Work out the finished part from the listing and answer in its coordinate system (mm). A direction names the side the tool comes from. Give positions to 0.01 mm unless a question says otherwise; leave off trailing zeros. Loops run counter-clockwise (first coordinate to the right, second up) from the corner with the lowest first, then second, coordinate; pieces in that order, holes last. Notation, with made-up numbers: (57, -21.75) - (80, -21.75) arc R16 cw to (80, -6.75) - close; hole circle Ø9 at (74.5, -7). An arc over 180 degrees is marked (long way). Use CSV: the item, a comma, the result in double quotes.
from build123d import *

# Parameters (mm, degrees)
BOSS_EXTRUDE1_DEPTH = 11.5
SKETCH4_R           = 4.5
CUT_EXTRUDE2_DEPTH  = 5
SKETCH5_R           = 2.75
CUT_EXTRUDE3_DEPTH  = 89.726115198
SKETCH6_R           = 2.5
CUT_EXTRUDE4_DEPTH  = 50.330582837
CUT_EXTRUDE5_DEPTH  = 8.2
CUT_EXTRUDE6_DEPTH  = 9
FILLET1_R           = 5.05
FILLET2_R           = 5
BOSS_EXTRUDE2_DEPTH = 18
SKETCH3_R           = 2.5
CUT_EXTRUDE1_DEPTH  = 4


with BuildPart() as part:
    # Sketch1 → Boss-Extrude1 (new body)
    with BuildSketch(Plane(origin=(0, 0, 0), x_dir=(1, 0, 0), z_dir=(0, 1, 0))):
        with BuildLine():
            Line((48.493420768, -25), (75.993420768, -25))
            ThreePointArc((75.993420768, -25), (79.695575847, 6.97245942), (70.497705508, 37.816312856))
            Line((70.497705508, 37.816312856), (43.415492301, 33.04098797))
            ThreePointArc((43.415492301, 33.04098797), (54.350723514, 4.755072162), (48.493420768, -25))
        make_face()
    extrude(amount=BOSS_EXTRUDE1_DEPTH)

    # Sketch4 → Cut-Extrude2 (cut)
    with BuildSketch(Plane.XZ):
        with Locations(Location((73.026415161, 17, 0), (0, 0, 270))):
            Circle(SKETCH4_R)
        with Locations(Location((68.964960805, -29.422635715, 0), (0, 0, 270))):
            Circle(SKETCH4_R)
    extrude(amount=-CUT_EXTRUDE2_DEPTH, mode=Mode.SUBTRACT)

    # Sketch5 → Cut-Extrude3 (cut, through all)
    with BuildSketch(Plane.XZ.offset(-5)):
        with Locations(Location((73.026415161, 17, 0), (0, 0, 270))):
            Circle(SKETCH5_R)
        with Locations(Location((68.964960805, -29.422635715, 0), (0, 0, 270))):
            Circle(SKETCH5_R)
    extrude(amount=-CUT_EXTRUDE3_DEPTH, mode=Mode.SUBTRACT)

    # Sketch6 → Cut-Extrude4 (cut, through all)
    with BuildSketch(Plane(origin=(45.954456534, 0, -4.020493985), x_dir=(0.08715574274765857, 0, 0.9961946980917455), z_dir=(-0.9961946980917455, 0, 0.08715574274765857))):
        with Locations((0, 7.5)):
            Circle(SKETCH6_R)
    extrude(amount=-CUT_EXTRUDE4_DEPTH, mode=Mode.SUBTRACT)

    # Sketch8 → Cut-Extrude5 (cut)
    with BuildSketch(Plane(origin=(79.695575847, 0, -6.97245942), x_dir=(-0.08715574274765857, 0, -0.9961946980917455), z_dir=(0.9961946980917455, 0, -0.08715574274765857))):
        with BuildLine():
            Line((-4.5, 7.5), (-4.5, 11.5))
            Line((-4.5, 11.5), (4.5, 11.5))
            Line((4.5, 11.5), (4.5, 7.5))
            ThreePointArc((4.5, 7.5), (0, 3), (-4.5, 7.5))
        make_face()
    extrude(amount=-CUT_EXTRUDE5_DEPTH, mode=Mode.SUBTRACT)

    # Sketch7 → Cut-Extrude6 (cut)
    with BuildSketch(Plane(origin=(0, 11.5, 0), x_dir=(1, 0, 0), z_dir=(0, 1, 0))):
        Polygon((51.16274886, 9.5454507), (52.043021862, -0.516115751), (60.012579447, 0.181130191), (59.132306445, 10.242696642), align=None)
    extrude(amount=-CUT_EXTRUDE6_DEPTH, mode=Mode.SUBTRACT)

    # Fillet1
    # the kernel refuses this fillet: 5.05 mm, written as the material it adds along each edge
    with BuildSketch(Plane(origin=(41.980572745, 2.5, 1.396465976), x_dir=(0, 1, 0), z_dir=(0.9961946980917454, 0, -0.08715574274765918))) as fillet1_piece_1_section:
        with BuildLine():
            CenterArc((FILLET1_R, -FILLET1_R), FILLET1_R, 90, 90)
            Line((0, -FILLET1_R), (0, 0))
            Line((0, 0), (FILLET1_R, 0))
        make_face()
    fillet1_piece_1 = extrude(amount=30.725886038, mode=Mode.PRIVATE)
    fillet1_piece_1 = fillet1_piece_1 - Plane(origin=(0, 3.651800065, 0), x_dir=(0.7957627874759549, 0, -0.6056084428642803), z_dir=(0, -1, 0)) * Cylinder(54.558334448, 82, mode=Mode.PRIVATE)
    add(fillet1_piece_1)
    with BuildSketch(Plane(origin=(71.709264508, 2.5, -11.343037894), x_dir=(0.08715574274765941, 0, 0.9961946980917454), z_dir=(-0.9961946980917455, 0, 0.08715574274765941))) as fillet1_piece_2_section:
        with BuildLine():
            CenterArc((FILLET1_R, FILLET1_R), FILLET1_R, 180, 90)
            Line((0, FILLET1_R), (0, 0))
            Line((0, 0), (FILLET1_R, 0))
        make_face()
    fillet1_piece_2 = extrude(amount=30.725886038, mode=Mode.PRIVATE)
    fillet1_piece_2 = fillet1_piece_2 - Plane(origin=(0, 3.643295327, 0), x_dir=(0.7957627874759549, 0, -0.6056084428642803), z_dir=(0, -1, 0)) * Cylinder(54.558334448, 82, mode=Mode.PRIVATE)
    add(fillet1_piece_2)

    # Fillet2
    fillet2_edges = [part.edges().sort_by_distance(p)[0] for p in [
        (48.493420768, 5.75, 25),
        (43.415492301, 5.75, -33.04098797),
    ]]
    fillet(fillet2_edges, radius=FILLET2_R)

    # Sketch2 → Boss-Extrude2 (add)
    with BuildSketch(Plane.XZ.offset(-11.5)):
        with BuildLine():
            Line((62.599920128, 13.5), (68.685879189, 13.5))
            ThreePointArc((68.685879189, 13.5), (67.280837144, 19.320687184), (65.383484153, 25))
            Line((65.383484153, 25), (58.599920128, 25))
            Line((58.599920128, 25), (58.599920128, 17.5))
            ThreePointArc((58.599920128, 17.5), (59.771493003, 14.671572875), (62.599920128, 13.5))
        make_face()
        with BuildLine():
            Line((54.670812559, -27.409905019), (53.368451226, -34.795963167))
            Line((53.368451226, -34.795963167), (60.048957671, -35.973916698))
            ThreePointArc((60.048957671, -35.973916698), (62.903687928, -30.710357294), (65.29813595, -25.222082418))
            Line((65.29813595, -25.222082418), (59.304636281, -24.165266718))
            ThreePointArc((59.304636281, -24.165266718), (56.315737825, -24.827889553), (54.670812559, -27.409905019))
        make_face()
    extrude(amount=-BOSS_EXTRUDE2_DEPTH)

    # Sketch3 → Cut-Extrude1 (cut)
    with BuildSketch(Plane(origin=(0, 29.5, 0), x_dir=(1, 0, 0), z_dir=(0, 1, 0))):
        with Locations(Location((58.610043571, 28.10449773, 0), (0, 0, 270))):
            Circle(SKETCH3_R)
        with Locations(Location((62.599920128, -17.5, 0), (0, 0, 270))):
            Circle(SKETCH3_R)
    extrude(amount=-CUT_EXTRUDE1_DEPTH, mode=Mode.SUBTRACT)


solid = part.part
Item 1: Given P1, Ø8, axis at y = 12, z = -29, coming from the +X side; P2, Ø1.8, axis at x = 64.5, y = 21, coming from the -Z side; P3, Ø10, axis at x = 59.5, z = -21.5, coming from the +Y side; P4, Ø4, axis at x = 58, y = 6.5, coming from the -Z side, each flat-ended and moving along its own axis, determine where each tip first touches the part or whether it passes through.
Determined:
P1,"stops at x = 75.98"
P2,"stops at z = -29.24"
P3,"stops at y = 29.5"
P4,"stops at z = -35.97"
Item 2: A cutting plane is placed at A-A on y = 17.5. Determine the outline of the cut face in (x, z).
Determined:
outline,"(53.37, -34.8) - (60.05, -35.97) arc R70 ccw to (65.3, -25.22) - (59.3, -24.17) arc R4 ccw to (54.67, -27.41) - close; (58.6, 17.5) arc R4 ccw to (62.6, 13.5) - (68.69, 13.5) arc R70 ccw to (65.38, 25) - (58.6, 25) - close"
Item 3: The mould has two halves that part along Z. Classify faces 6 (the cylindrical face through (62.867, 20.374, -30.786)), 7 (the flat face through (64, 11, 25)), 8 (the cylindrical face through (56.392, 27.528, -26.951)): pulls with the +Z half, pulls with the -Z half, needs draft (parallel to the pull), parting line crosses it, or undercut.
Determined:
face 6,"pulls with the -Z half"
face 7,"pulls with the +Z half"
face 8,"undercut"
Item 4: A cutting plane is placed at C-C on z = 7.5. Determine the outline of the cut face in (x, y), and give its area (3 significant figures).
Determined:
outline,"(54.04, 0) - (79.65, 0) - (79.65, 11.5) - (54.04, 11.5) - close"
area,"294 mm²"
Item 5: For faces 1 (the flat face through (58.6, 20, 21)), 2 (the flat face through (67, 5, -27)), 3 (the cylindrical face through (59.741, 20.374, 14.703)), 4 (the cylindrical face through (67.304, 20.374, 19.24)), 5 (the flat face through (62.34, 20.37, -24.7)), determine the directions among +Z, -Z, +X, -X, +Y, -Y from which every point of the face is accessible in a straight line to the end or side of a thin tool.
Determined:
face 1,"+Z, -X, +Y"
face 2,"-Y"
face 3,"-X, +Y"
face 4,"+Z, +X, +Y"
face 5,"+X, +Y"
Item 6: Find the intervals of material crossed by line 1 (Z direction, x = 69, y = 3.25); line 2 (Y direction, x = 60, z = -14); line 3 (Y direction, x = 63, z = -5.5), in increasing order.
Determined:
line 1,"z = -37.55 to -33.92, -24.92 to 14.99, 19.01 to 25"
line 2,"y = 0 to 11.5"
line 3,"y = 0 to 5, 10 to 11.5"
Item 7: A cutting plane is placed at B-B on y = 6. Determine the outline of the cut face in (x, z).
Determined:
outline,"(47.43, -26.97) arc R5 ccw to (50.91, -34.36) - (70.5, -37.82) arc R80 ccw to (79.21, -11.19) - (71.16, -10.48) - (71.35, -8.25) - (59.4, -7.2) - (59.15, -10) - (53.72, -9.52) arc R54.56 cw to start; (51.39, 18.32) arc R54.56 cw to (54.56, 0.05) - (59.99, -0.42) - (59.75, -3.22) - (71.7, -4.27) - (71.9, -2.03) - (79.95, -2.74) arc R80 ccw to (75.99, 25) - (56.1, 25) arc R5 ccw to start; hole circle Ø5.5 at (68.96, -29.42); hole circle Ø5.5 at (73.03, 17)"
